Work out the finished part from the listing and answer in its coordinate system (mm). A direction names the side the tool comes from. Round coordinates to 2 decimals unless told otherwise and drop trailing zeros. Loops run counter-clockwise (first coordinate to the right, second up) from the corner with the lowest first, then second, coordinate; pieces in that order, holes last.
```python
from build123d import *

# Parameters (mm, degrees)
F1_DEPTH  = 20
F3_W      = 195
F3_H      = 125
F4_DEPTH  = 10
F5_W      = 20
F5_H      = 73
F6_DEPTH  = 5
F7_R      = 3
F8_DEPTH  = 20.001
F9_R      = 3
F10_DEPTH = 10.001
F12_W     = 15
F12_H     = 20
F13_DEPTH = 1.5


with BuildPart() as f1:
    # F0 (on Front) → F1 (new body)
    with BuildSketch(Plane.XZ):
        Polygon((0, 10), (0, 0), (110, 0), (110, 10), (85, 10), (85, 53), (172.5, 53), (172.5, 218), (-62.5, 218), (-62.5, 53), (25, 53), (25, 10), align=None)
    extrude(amount=F1_DEPTH)

    # F3 (on face) → F4 (cut)
    with BuildSketch(Plane.XZ.offset(20)):
        with Locations((55, 135.5)):
            Rectangle(F3_W, F3_H)
    extrude(amount=-F4_DEPTH, mode=Mode.SUBTRACT)

    # F5 (on face) → F6 (cut)
    with BuildSketch(Plane.XZ.offset(20)):
        with Locations((55, 36.5)):
            Rectangle(F5_W, F5_H)
    extrude(amount=-F6_DEPTH, mode=Mode.SUBTRACT)

    # F7 (on face) → F8 (cut, through all)
    with BuildSketch(Plane.XZ.offset(20)):
        with Locations((-52.5, 208)):
            Circle(F7_R)
        with Locations((162.5, 208)):
            Circle(F7_R)
        with Locations((162.5, 63)):
            Circle(F7_R)
        with Locations((-52.5, 63)):
            Circle(F7_R)
        with Locations((35, 10)):
            Circle(F7_R)
        with Locations((35, 43)):
            Circle(F7_R)
        with Locations((75, 43)):
            Circle(F7_R)
        with Locations((75, 10)):
            Circle(F7_R)
    extrude(amount=-F8_DEPTH, mode=Mode.SUBTRACT)

    # F9 (on face) → F10 (cut, through all)
    with BuildSketch(Plane.XY.offset(10)):
        with Locations((10, -10)):
            Circle(F9_R)
        with Locations((100, -10)):
            Circle(F9_R)
    extrude(amount=-F10_DEPTH, mode=Mode.SUBTRACT)

    # F12 (on face) → F13 (cut)
    with BuildSketch(Plane.XZ.offset(20)):
        with Locations((-12.5, 208)):
            Rectangle(F12_W, F12_H)
        with Locations((32.5, 208)):
            Rectangle(F12_W, F12_H)
        with Locations((77.5, 208)):
            Rectangle(F12_W, F12_H)
        with Locations((122.5, 208)):
            Rectangle(F12_W, F12_H)
    extrude(amount=-F13_DEPTH, mode=Mode.SUBTRACT)


solid = f1.part
```
1. Determine the mould class of faces 6 (the face through (72.79, -10.14, 45.03)), 7 (the face through (97, -10, 5)) for opening direction Z: +Z half, -Z half, draft (parallel to the pull), parting line (faces both ways), or undercut.
Answer key:
face 6: undercut
face 7: draft
2. Find section A-A (x = 93). Write down the section's boundary in (y, z).
Answer key:
outline: (-20, 0) - (0, 0) - (0, 10) - (-20, 10) - close; (-20, 53) - (0, 53) - (0, 218) - (-20, 218) - (-20, 198) - (-10, 198) - (-10, 73) - (-20, 73) - close
3. Find section C-C (x = 10). Write down the section's boundary in (y, z), then the cut area to 3 significant figures.
Answer key:
outline: (-20, 0) - (-13, 0) - (-13, 10) - (-20, 10) - close; (-20, 53) - (0, 53) - (0, 218) - (-20, 218) - (-20, 198) - (-10, 198) - (-10, 73) - (-20, 73) - close; (-7, 0) - (0, 0) - (0, 10) - (-7, 10) - close
area: 2,190 mm2
4. Find section D-D (z = 32). Write down the section's boundary in (x, y).
Answer key:
outline: (25, -20) - (45, -20) - (45, -15) - (65, -15) - (65, -20) - (85, -20) - (85, 0) - (25, 0) - close
5. Consider probe 1 along Z at (x, y) = (75, -7.25); probe 2 along Z at (x, y) = (162.5, -13.75); probe 3 along X at (y, z) = (-15.5, 87). Determine where each line is inside the solid, lowest interval first.
Answer key:
probe 1: z = 0 to 7, 13 to 40, 46 to 218
probe 2: z = 53 to 60, 66 to 205, 211 to 218
probe 3: x = -62.5 to -42.5, 152.5 to 172.5
6. Given pin 1 (8 mm diameter, centred on x = 35, z = 10, fed in from -Y); pin 2 (12 mm diameter, centred on x = 123, z = 207.5, fed in from -Y); pin 3 (1.5 mm diameter, centred on x = 140, y = -8.5, fed in from -Z); pin 4 (10 mm diameter, centred on x = 52.5, z = 44.5, fed in from -Y), each flat-ended and moving along its own axis, determine where each tip first touches the part or whether it passes through.
Answer key:
pin 1: stops at y = -20
pin 2: stops at y = -18.5
pin 3: stops at z = 53
pin 4: stops at y = -15
7. Which of the six approach directions +Z, -Z, +X, -X, +Y, -Y give full straight-line access (tool end or side, diameter ignored) to faces 1 (the face through (32, -18.5, 208)), 2 (the face through (54, -10, 136)), 3 (the face through (11.61, -7.47, 5.07)), 4 (the face through (25, -10, 32)), 5 (the face through (0, -10, 5))?
Answer key:
face 1: +Z, -Y
face 2: -Y
face 3: -Z
face 4: -X, +Y, -Y
face 5: -Z, -X, +Y, -Y
8. Find section B-B (z = 208). Write down the section's boundary in (x, y), then the cut area to 3 significant figures.
Answer key:
outline: (-62.5, -20) - (-55.5, -20) - (-55.5, 0) - (-62.5, 0) - close; (-49.5, -20) - (-20, -20) - (-20, -18.5) - (-5, -18.5) - (-5, -20) - (25, -20) - (25, -18.5) - (40, -18.5) - (40, -20) - (70, -20) - (70, -18.5) - (85, -18.5) - (85, -20) - (115, -20) - (115, -18.5) - (130, -18.5) - (130, -20) - (159.5, -20) - (159.5, 0) - (-49.5, 0) - close; (165.5, -20) - (172.5, -20) - (172.5, 0) - (165.5, 0) - close
area: 4,370 mm2
